CAD build for the part. Positions are in the model's coordinates, mm. Coordinates: 2 decimals unless noted, no trailing zeros. Order: outer loops, then holes, each group sorted by start corner. A loop starts at its lowest first (then second) coordinate and runs counter-clockwise, first axis right, second up. Notation, with made-up numbers: M -12,-31 L 8,-31 A12 ccw 8,-9 Z; hole C 76.5,37 d4. An arc over 180 degrees is marked long. Write item = value, one per line.
from build123d import *

# Parameters (mm, degrees)
SKETCH1_R           = 2.55
BOSS_EXTRUDE1_DEPTH = 3


with BuildPart() as part:
    # Sketch1 → Boss-Extrude1 (new body)
    with BuildSketch(Plane(origin=(0, 0, 0), x_dir=(1, 0, 0), z_dir=(0, 1, 0))):
        with BuildLine():
            Line((-19.389943983, 28.212319901), (10.610056017, 28.212319901))
            ThreePointArc((10.610056017, 28.212319901), (12.731376361, 27.333640245), (13.610056017, 25.212319901))
            Line((13.610056017, 25.212319901), (13.610056017, 10.212319901))
            ThreePointArc((13.610056017, 10.212319901), (14.488735674, 8.090999558), (16.610056017, 7.212319901))
            Line((16.610056017, 7.212319901), (32.610056017, 7.212319901))
            Line((32.610056017, 7.212319901), (42.610056017, 7.212319901))
            ThreePointArc((42.610056017, 7.212319901), (44.731376361, 6.333640245), (45.610056017, 4.212319901))
            Line((45.610056017, 4.212319901), (45.610056017, -46.787680099))
            ThreePointArc((45.610056017, -46.787680099), (44.145589923, -50.323214005), (40.610056017, -51.787680099))
            Line((40.610056017, -51.787680099), (-49.389943983, -51.787680099))
            ThreePointArc((-49.389943983, -51.787680099), (-52.925477889, -50.323214005), (-54.389943983, -46.787680099))
            Line((-54.389943983, -46.787680099), (-54.389943983, 4.212319901))
            ThreePointArc((-54.389943983, 4.212319901), (-53.511264326, 6.333640245), (-51.389943983, 7.212319901))
            Line((-51.389943983, 7.212319901), (-41.389943983, 7.212319901))
            Line((-41.389943983, 7.212319901), (-25.389943983, 7.212319901))
            ThreePointArc((-25.389943983, 7.212319901), (-23.268623639, 8.090999558), (-22.389943983, 10.212319901))
            Line((-22.389943983, 10.212319901), (-22.389943983, 25.212319901))
            ThreePointArc((-22.389943983, 25.212319901), (-21.511264326, 27.333640245), (-19.389943983, 28.212319901))
        make_face()
        with Locations((-10.389943983, 18.212319901)):
            Circle(SKETCH1_R, mode=Mode.SUBTRACT)
        with Locations((1.610056017, 18.212319901)):
            Circle(SKETCH1_R, mode=Mode.SUBTRACT)
        with Locations((-4.389943983, -41.787680099)):
            Circle(SKETCH1_R, mode=Mode.SUBTRACT)
        with Locations((-4.389943983, -21.787680099)):
            Circle(SKETCH1_R, mode=Mode.SUBTRACT)
        with Locations((-28.469943983, -22.787680099)):
            Circle(SKETCH1_R, mode=Mode.SUBTRACT)
        with Locations((19.690056017, -22.787680099)):
            Circle(SKETCH1_R, mode=Mode.SUBTRACT)
        with BuildLine():
            Line((40.110056017, -38.787680099), (40.110056017, -40.287680099))
            ThreePointArc((40.110056017, -40.287680099), (38.610056017, -41.787680099), (37.110056017, -40.287680099))
            Line((37.110056017, -40.287680099), (37.110056017, -38.787680099))
            ThreePointArc((37.110056017, -38.787680099), (38.610056017, -37.287680099), (40.110056017, -38.787680099))
        make_face(mode=Mode.SUBTRACT)
        with BuildLine():
            Line((37.110056017, -46.787680099), (37.110056017, -45.287680099))
            ThreePointArc((37.110056017, -45.287680099), (38.610056017, -43.787680099), (40.110056017, -45.287680099))
            Line((40.110056017, -45.287680099), (40.110056017, -46.787680099))
            ThreePointArc((40.110056017, -46.787680099), (38.610056017, -48.287680099), (37.110056017, -46.787680099))
        make_face(mode=Mode.SUBTRACT)
        with BuildLine():
            Line((41.160056017, -19.229266089), (41.160056017, -29.229266089))
            ThreePointArc((41.160056017, -29.229266089), (38.610056017, -31.779266089), (36.060056017, -29.229266089))
            Line((36.060056017, -29.229266089), (36.060056017, -19.229266089))
            ThreePointArc((36.060056017, -19.229266089), (38.610056017, -16.679266089), (41.160056017, -19.229266089))
        make_face(mode=Mode.SUBTRACT)
        with BuildLine():
            Line((-45.889943983, -38.787680099), (-45.889943983, -40.287680099))
            ThreePointArc((-45.889943983, -40.287680099), (-47.389943983, -41.787680099), (-48.889943983, -40.287680099))
            Line((-48.889943983, -40.287680099), (-48.889943983, -38.787680099))
            ThreePointArc((-48.889943983, -38.787680099), (-47.389943983, -37.287680099), (-45.889943983, -38.787680099))
        make_face(mode=Mode.SUBTRACT)
        with BuildLine():
            Line((-48.889943983, -46.787680099), (-48.889943983, -45.287680099))
            ThreePointArc((-48.889943983, -45.287680099), (-47.389943983, -43.787680099), (-45.889943983, -45.287680099))
            Line((-45.889943983, -45.287680099), (-45.889943983, -46.787680099))
            ThreePointArc((-45.889943983, -46.787680099), (-47.389943983, -48.287680099), (-48.889943983, -46.787680099))
        make_face(mode=Mode.SUBTRACT)
        with BuildLine():
            Line((-44.839943983, -19.229266089), (-44.839943983, -29.229266089))
            ThreePointArc((-44.839943983, -29.229266089), (-47.389943983, -31.779266089), (-49.939943983, -29.229266089))
            Line((-49.939943983, -29.229266089), (-49.939943983, -19.229266089))
            ThreePointArc((-49.939943983, -19.229266089), (-47.389943983, -16.679266089), (-44.839943983, -19.229266089))
        make_face(mode=Mode.SUBTRACT)
    extrude(amount=BOSS_EXTRUDE1_DEPTH)


solid = part.part
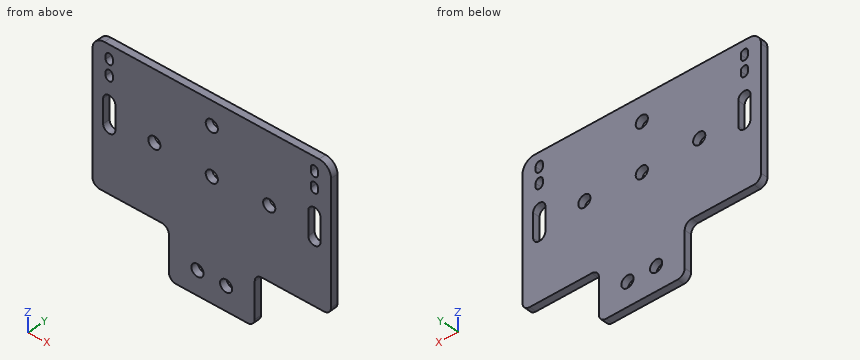
(1) Slice it at C-C, the plane x = 39. Write the cut outline in (y, z).
Evaluation:
outline = M 0,-7.21 L 3,-7.21 L 3,16.71 L 0,16.71 Z; M 0,31.75 L 3,31.75 L 3,37.34 L 0,37.34 Z; M 0,41.74 L 3,41.74 L 3,43.84 L 0,43.84 Z; M 0,48.24 L 3,48.24 L 3,51.79 L 0,51.79 Z
(2) Slice it at D-D, the plane y = 1.85. State how many separate pieces and enclosed holes the cut face has, then the cut area to 3 significant figures.
Evaluation:
separate_pieces = 1
enclosed_holes = 12
area = 6,330 mm²
(3) Wall check: line 1 (X direction, y = 1.2, z = 26); line 2 (X direction, y = 0.6, z = 39); line 3 (Z direction, x = -6, y = 0.1). Give the ranges that are in metal, low to high. Write a range as from..to.
Evaluation:
line_1 = -54.39..-49.94, -44.84..36.06, 41.16..45.61
line_2 = -54.39..-48.89, -45.89..37.11, 40.11..45.61
line_3 = -28.21..19.81, 23.77..39.81, 43.77..51.79
(4) Slice it at A-A, the plane x = -29. Write the cut outline in (y, z).
Evaluation:
outline = M 0,-7.21 L 3,-7.21 L 3,20.29 L 0,20.29 Z; M 0,25.28 L 3,25.28 L 3,51.79 L 0,51.79 Z
(5) Slice it at B-B, the plane z = -12. Write the cut outline in (x, y).
Evaluation:
outline = M -22.39,0 L 13.61,0 L 13.61,3 L -22.39,3 Z
(6) Pin check, flat tips, straight feed: pin 1 Ø1.5 at (x, y) = (-33.5, 1.5) entering from -Z; pin 2 Ø3 at (x, z) = (-4.39, 41.79) entering from -Y. Stop position of each tip, or through.
Evaluation:
pin_1 = -7.21
pin_2 = through
